from build123d import *

# Parameters (mm, degrees)
ESQUISSE1_R        = 3.4
ESQUISSE1_R_2      = 22
BOSS_EXTRU_2_DEPTH = 5


with BuildPart() as part:
    # Esquisse1 → Boss.-Extru.2 (new body)
    with BuildSketch(Plane.XY):
        with BuildLine():
            ThreePointArc((44.919487431, -50), (48.51195232, -48.51195232), (50, -44.919487431))
            Line((50, -44.919487431), (50, -33.862050579))
            ThreePointArc((50, -33.862050579), (49.777389032, -32.945051), (49.159111773, -32.232185585))
            ThreePointArc((49.159111773, -32.232185585), (45.31641316, -26.748192273), (45.795558863, -20.069050512))
            ThreePointArc((45.795558863, -20.069050512), (48.937602838, -10.252366967), (50, 0))
            ThreePointArc((50, 0), (48.936869799, 10.255865358), (45.79268903, 20.075597908))
            ThreePointArc((45.79268903, 20.075597908), (45.313248124, 26.757056992), (49.158537806, 32.242082639))
            ThreePointArc((49.158537806, 32.242082639), (49.777227562, 32.955043184), (50, 33.872355669))
            Line((50, 33.872355669), (50, 44.919487431))
            ThreePointArc((50, 44.919487431), (48.51195232, 48.51195232), (44.919487431, 50))
            Line((44.919487431, 50), (33.862050579, 50))
            ThreePointArc((33.862050579, 50), (32.945051, 49.777389032), (32.232185585, 49.159111773))
            ThreePointArc((32.232185585, 49.159111773), (26.748192273, 45.31641316), (20.069050512, 45.795558863))
            ThreePointArc((20.069050512, 45.795558863), (10.252366967, 48.937602838), (0, 50))
            ThreePointArc((0, 50), (-10.255865358, 48.936869799), (-20.075597908, 45.79268903))
            ThreePointArc((-20.075597908, 45.79268903), (-26.757056992, 45.313248124), (-32.242082639, 49.158537806))
            ThreePointArc((-32.242082639, 49.158537806), (-32.955043184, 49.777227562), (-33.872355669, 50))
            Line((-33.872355669, 50), (-44.919487431, 50))
            ThreePointArc((-44.919487431, 50), (-48.51195232, 48.51195232), (-50, 44.919487431))
            Line((-50, 44.919487431), (-50, 33.862050579))
            ThreePointArc((-50, 33.862050579), (-49.777389032, 32.945051), (-49.159111773, 32.232185585))
            ThreePointArc((-49.159111773, 32.232185585), (-45.31641316, 26.748192273), (-45.795558863, 20.069050512))
            ThreePointArc((-45.795558863, 20.069050512), (-48.937602838, 10.252366967), (-50, 0))
            ThreePointArc((-50, 0), (-48.936869799, -10.255865358), (-45.79268903, -20.075597908))
            ThreePointArc((-45.79268903, -20.075597908), (-45.313248124, -26.757056992), (-49.158537806, -32.242082639))
            ThreePointArc((-49.158537806, -32.242082639), (-49.777227562, -32.955043184), (-50, -33.872355669))
            Line((-50, -33.872355669), (-50, -44.919487431))
            ThreePointArc((-50, -44.919487431), (-48.51195232, -48.51195232), (-44.919487431, -50))
            Line((-44.919487431, -50), (-33.862050579, -50))
            ThreePointArc((-33.862050579, -50), (-32.945051, -49.777389032), (-32.232185585, -49.159111773))
            ThreePointArc((-32.232185585, -49.159111773), (-26.748192273, -45.31641316), (-20.069050512, -45.795558863))
            ThreePointArc((-20.069050512, -45.795558863), (-10.252366967, -48.937602838), (0, -50))
            ThreePointArc((0, -50), (10.255865358, -48.936869799), (20.075597908, -45.79268903))
            ThreePointArc((20.075597908, -45.79268903), (26.757056992, -45.313248124), (32.242082639, -49.158537806))
            ThreePointArc((32.242082639, -49.158537806), (32.955043184, -49.777227562), (33.872355669, -50))
            Line((33.872355669, -50), (44.919487431, -50))
        make_face()
        with Locations((-40, -40)):
            Circle(ESQUISSE1_R, mode=Mode.SUBTRACT)
        with BuildLine():
            ThreePointArc((-29.746951128, -33.282485034), (-33.282485092, -33.282485209), (-33.28248515, -29.746951244))
            Line((-33.28248515, -29.746951244), (-22.675883316, -19.14034941))
            ThreePointArc((-22.675883316, -19.14034941), (-19.14034941, -19.14034941), (-19.14034941, -22.675883316))
            Line((-19.14034941, -22.675883316), (-29.746951128, -33.282485034))
        make_face(mode=Mode.SUBTRACT)
        with Locations((40, -40)):
            Circle(ESQUISSE1_R, mode=Mode.SUBTRACT)
        with BuildLine():
            ThreePointArc((33.282485034, -29.746951128), (33.282485209, -33.282485092), (29.746951244, -33.28248515))
            Line((29.746951244, -33.28248515), (19.14034941, -22.675883316))
            ThreePointArc((19.14034941, -22.675883316), (19.14034941, -19.14034941), (22.675883316, -19.14034941))
            Line((22.675883316, -19.14034941), (33.282485034, -29.746951128))
        make_face(mode=Mode.SUBTRACT)
        Circle(ESQUISSE1_R_2, mode=Mode.SUBTRACT)
        with BuildLine():
            ThreePointArc((-33.282485034, 29.746951128), (-33.282485209, 33.282485092), (-29.746951244, 33.28248515))
            Line((-29.746951244, 33.28248515), (-19.14034941, 22.675883316))
            ThreePointArc((-19.14034941, 22.675883316), (-19.14034941, 19.14034941), (-22.675883316, 19.14034941))
            Line((-22.675883316, 19.14034941), (-33.282485034, 29.746951128))
        make_face(mode=Mode.SUBTRACT)
        with Locations((-40, 40)):
            Circle(ESQUISSE1_R, mode=Mode.SUBTRACT)
        with BuildLine():
            ThreePointArc((29.746951128, 33.282485034), (33.282485092, 33.282485209), (33.28248515, 29.746951244))
            Line((33.28248515, 29.746951244), (22.675883316, 19.14034941))
            ThreePointArc((22.675883316, 19.14034941), (19.14034941, 19.14034941), (19.14034941, 22.675883316))
            Line((19.14034941, 22.675883316), (29.746951128, 33.282485034))
        make_face(mode=Mode.SUBTRACT)
        with Locations((40, 40)):
            Circle(ESQUISSE1_R, mode=Mode.SUBTRACT)
    extrude(amount=BOSS_EXTRU_2_DEPTH)


solid = part.part
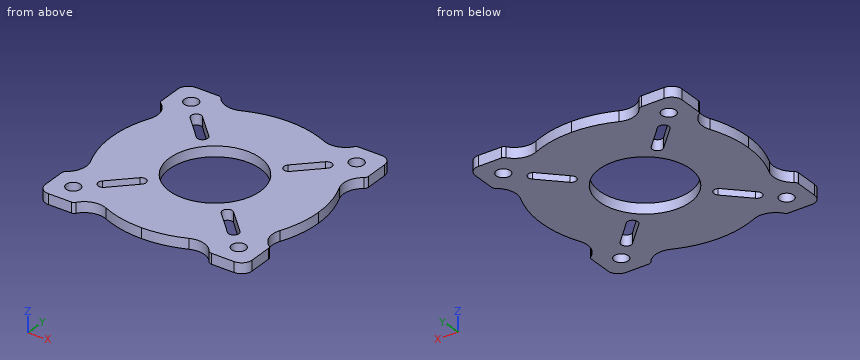
Model file for the job. Use its own axes, mm. Give positions to 0.01 mm unless a question says otherwise; leave off trailing zeros. Write each loop counter-clockwise with the first axis right and the second up, starting at its lowest first coordinate (ties: lowest second). Pieces come first, ordered by that corner, then holes. Notation, with made-up numbers: M -36.75,40.25 L -12.75,40.25 A9 cw -12.75,55.25 Z; hole C -26,41 d11. An arc over 180 degrees is marked long. One line per item, written item: value. Start each with the question number.
Q1. Drop flat-ended pins along their axis: pin 1 Ø3 at (x, y) = (20.5, -36.5) entering from -Z; pin 2 Ø1 at (x, z) = (-5.5, 4) entering from +Y; pin 3 Ø3 at (x, z) = (31, 3.5) entering from -Y; pin 4 Ø2 at (y, z) = (-28, 4.5) entering from +X. Give the stop position or say it passes through.
Q2. Probe probe 1 along Y at (x, z) = (-40.5, 3.1); probe 2 along Y at (x, z) = (-41.5, 1.9); probe 3 along X at (y, z) = (37, 1.6). List the from-to ranges inside material, lowest first. Write a range as [from, to].
Q3. Saw through at C-C, the plane x = 11.5. Write the cut outline in (y, z) (3 decimals), plus the area to 3 significant figures.
Q4. Saw through at A-A, the plane y = 40. Write the cut outline in (x, z).
Q5. Saw through at D-D, the plane y = 4. Write the cut outline in (x, z).
Output values:
1. pin 1: stops at z = 0
1. pin 2: stops at y = 49.75
1. pin 3: stops at y = -49.45
1. pin 4: stops at x = 46.25
2. probe 1: y = [-50, -43.36], [-36.64, 36.64], [43.36, 50]
2. probe 2: y = [-50, -43.05], [-36.95, 36.95], [43.05, 50]
2. probe 3: x = [-50, -41.6], [-38.4, 38.4], [41.6, 50]
3. outline: M -48.66,0 L -18.755,0 L -18.755,5 L -48.66,5 Z; M 18.755,0 L 48.66,0 L 48.66,5 L 18.755,5 Z
3. area: 299 mm²
4. outline: M -50,0 L -43.4,0 L -43.4,5 L -50,5 Z; M -36.6,0 L 36.6,0 L 36.6,5 L -36.6,5 Z; M 43.4,0 L 50,0 L 50,5 L 43.4,5 Z
5. outline: M -49.84,0 L -21.63,0 L -21.63,5 L -49.84,5 Z; M 21.63,0 L 49.84,0 L 49.84,5 L 21.63,5 Z
